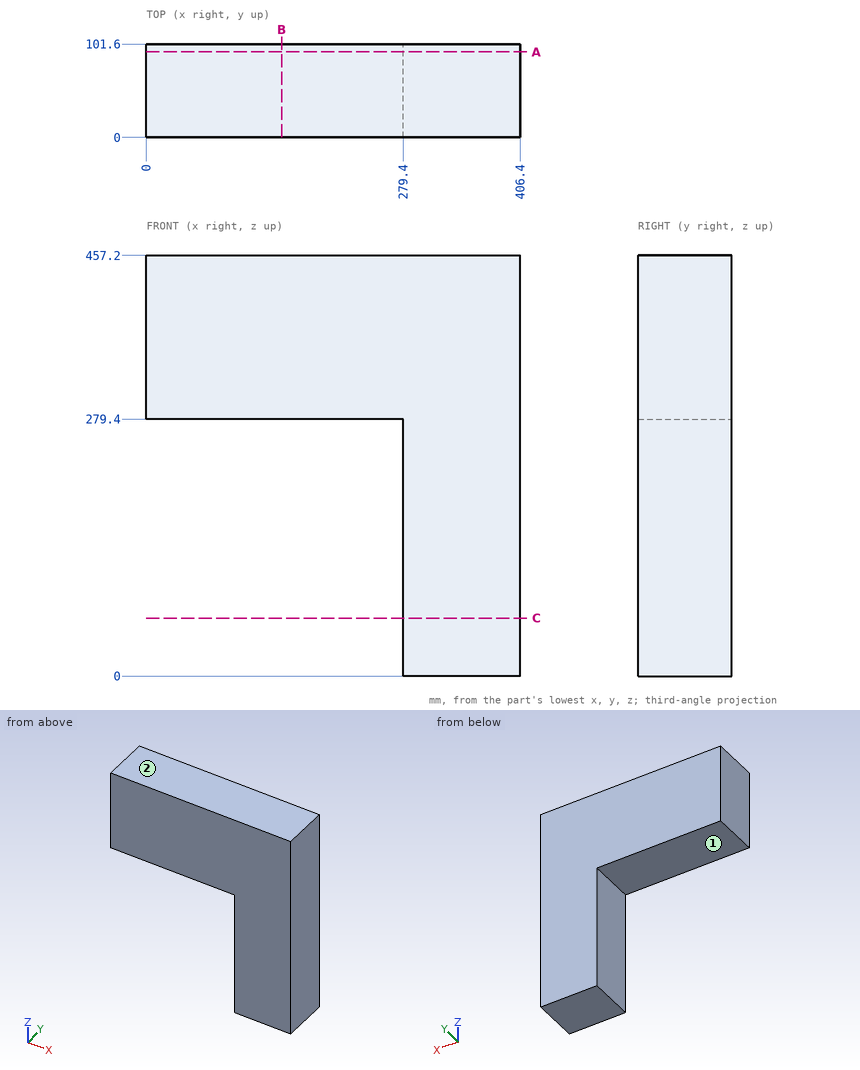
Source: three-view drawing plus pictorial views. Frame: mm from the lowest corner of the part. A direction names the side the tool comes from. Give positions to 0.01 mm unless a question says otherwise; leave off trailing zeros. Order: outer loops, then holes, each group sorted by start corner. A loop starts at its lowest first (then second) coordinate and runs counter-clockwise, first axis right, second up. Notation, with made-up numbers: M 37,13.25 L 46,13.25 A33 cw 46,49.25 Z; hole C 40,-32.5 d3. An arc over 180 degrees is marked long. One line per question, with ' | ' between items. Start each with the question number.
1. Access query for the marked faces 1 and 2. Directions: +Z, -Z, +X, -X, +Y, -Y. A direction counts if a zero-diameter tool reaches every point of the face in a straight line with its end or side. Return the directions, or none.
2. Material intervals for probe 1 along Z at (x, y) = (174, 74.5); probe 2 along X at (y, z) = (48, 56), sorted ascending. Write a range as [from, to].
3. Section query B-B (x = 147). Return the cut outline in (y, z), and give its area (3 significant figures).
4. First-contact query: pin 1 Ø1.5 at (y, z) = (58.5, 156.5) entering from -X. Flat tip, straight axial feed; report the tip coordinate or a pass-through.
5. Section query A-A (y = 93). Return the cut outline in (x, z).
6. Section query C-C (z = 63). Return the cut outline in (x, y), and give its area (3 significant figures).
Here are the results:
1) face 1: -Z, -X, +Y, -Y | face 2: +Z, +X, -X, +Y, -Y
2) probe 1: [279.4, 457.2] | probe 2: [279.4, 406.4]
3) outline: M 0,279.4 L 101.6,279.4 L 101.6,457.2 L 0,457.2 Z | area: 18,100 mm²
4) pin 1: x = 279.4
5) outline: M 0,279.4 L 279.4,279.4 L 279.4,0 L 406.4,0 L 406.4,457.2 L 0,457.2 Z
6) outline: M 279.4,0 L 406.4,0 L 406.4,101.6 L 279.4,101.6 Z | area: 12,900 mm²
